```python
from build123d import *

# Parameters (mm, degrees)
F1_DEPTH = 25.4
F2_SIZE  = 5.08


with BuildPart() as f1:
    # F0 (on Front) → F1 (new body)
    with BuildSketch(Plane.XZ):
        Polygon((29.543495, 26.300911), (-39.631508, 19.095181), (-29.543485, -29.903777), (21.256905, -29.903777), align=None)
    extrude(amount=F1_DEPTH)

    # F2
    f2_edges = [f1.edges().sort_by_distance(p)[0] for p in [
        (29.543495, -12.7, 26.300911),
    ]]
    chamfer(f2_edges, length=F2_SIZE)


solid = f1.part
```
Here's how the part is built. I have some questions about the finished solid (model axes, mm). Round coordinates to 2 decimals unless told otherwise and drop trailing zeros. Order: outer loops, then holes, each group sorted by start corner. A loop starts at its lowest first (then second) coordinate and runs counter-clockwise, first axis right, second up. Notation, with made-up numbers: M 63,48.5 L 112,48.5 A20 ccw 112,56.5 Z; hole C 45,83.5 d2. An arc over 180 degrees is marked long. Answer in a Markdown table with one row per item.
Item 1: Imagine slicing it at C-C, the plane z = 0.5. Write out the boundary of the cut face in (x, y).
A:
| item | result |
|---|---|
| outline | M -35.8,-25.4 L 25.74,-25.4 L 25.74,0 L -35.8,0 Z |
Item 2: Imagine slicing it at B-B, the plane x = 15.5. Write out the boundary of the cut face in (y, z).
A:
| item | result |
|---|---|
| outline | M -25.4,-29.9 L 0,-29.9 L 0,24.84 L -25.4,24.84 Z |
Item 3: If I drill on L1, parallel to X at y = -7, z = 18; L2, parallel to X at y = -10.25, z = -10; L3, parallel to Z at x = 6.5, y = -4.5, over which ranges is the centre line in solid material (lowest first)? Write a range as from..to.
A:
| item | result |
|---|---|
| L1 | x = -39.41..28.32 |
| L2 | x = -33.64..24.19 |
| L3 | z = -29.9..23.9 |
Item 4: I'm going to push flat-ended pins straight in: pin 1 (12 mm diameter, centred on y = -10, z = -3, fed in from -X); pin 2 (3 mm diameter, centred on y = -6, z = -21, fed in from +X); pin 3 (5 mm diameter, centred on x = 18, y = -9, fed in from +Z). Where does each tip first touch, or does it pass through?
A:
| item | result |
|---|---|
| pin 1 | stops at x = -36.32 |
| pin 2 | stops at x = 22.79 |
| pin 3 | stops at z = 25.36 |
Item 5: Imagine slicing it at A-A, the plane y = -2. Write out the boundary of the cut face in (x, z).
A:
| item | result |
|---|---|
| outline | M -39.63,19.1 L -29.54,-29.9 L 21.26,-29.9 L 28.8,21.28 L 24.49,25.77 Z |
